from build123d import *

# Parameters (mm, degrees)
SKETCH1_W           = 42.3
SKETCH1_H           = 42.3
SKETCH1_R           = 1.5
SKETCH1_R_2         = 4.7625
BOSS_EXTRUDE1_DEPTH = 5.21
SKETCH2_R           = 0.75565
SKETCH2_R_2         = 1.1303
CUT_EXTRUDE1_DEPTH  = 6.21
CHAMFER1_SIZE       = 2
SKETCH4_R           = 6.96
SKETCH4_R_2         = 4.7625
BOSS_EXTRUDE2_DEPTH = 1.14
SKETCH5_R           = 4
SKETCH5_R_2         = 1.5
CUT_EXTRUDE2_DEPTH  = 2
FILLET1_R           = 5


with BuildPart() as part:
    # Sketch1 → Boss-Extrude1 (new body)
    with BuildSketch(Plane(origin=(0, 0, 0), x_dir=(1, 0, 0), z_dir=(0, 1, 0))):
        with Locations((21.15, 21.15)):
            Rectangle(SKETCH1_W, SKETCH1_H)
        with Locations((36.65, 36.65)):
            Circle(SKETCH1_R, mode=Mode.SUBTRACT)
        with Locations((5.65, 5.65)):
            Circle(SKETCH1_R, mode=Mode.SUBTRACT)
        with Locations((36.65, 5.65)):
            Circle(SKETCH1_R, mode=Mode.SUBTRACT)
        with Locations((5.65, 36.65)):
            Circle(SKETCH1_R, mode=Mode.SUBTRACT)
        with Locations((21.15, 21.15)):
            Circle(SKETCH1_R_2, mode=Mode.SUBTRACT)
    extrude(amount=BOSS_EXTRUDE1_DEPTH)

    # Sketch2 → Cut-Extrude1 (cut, through all)
    with BuildSketch(Plane(origin=(0, 5.21, 0), x_dir=(1, 0, 0), z_dir=(0, 1, 0))):
        with Locations((11.056075115, 23.854659021)):
            Circle(SKETCH2_R)
        with Locations((28.539265863, 28.539265863)):
            Circle(SKETCH2_R)
        with Locations((23.854659021, 11.056075115)):
            Circle(SKETCH2_R)
        with Locations((28.539265863, 13.760734137)):
            Circle(SKETCH2_R_2)
        with Locations((13.760734137, 28.539265863)):
            Circle(SKETCH2_R_2)
    extrude(amount=-CUT_EXTRUDE1_DEPTH, mode=Mode.SUBTRACT)

    # Chamfer1
    chamfer1_edges = [part.edges().sort_by_distance(p)[0] for p in [
        (35.15, 5.21, -36.65),
        (4.15, 5.21, -5.65),
        (35.15, 5.21, -5.65),
        (4.15, 5.21, -36.65),
    ]]
    chamfer(chamfer1_edges, length=CHAMFER1_SIZE)

    # Sketch4 → Boss-Extrude2 (add)
    with BuildSketch(Plane(origin=(0, 5.21, 0), x_dir=(1, 0, 0), z_dir=(0, 1, 0))):
        with Locations((21.15, 21.15)):
            Circle(SKETCH4_R)
        with Locations((21.15, 21.15)):
            Circle(SKETCH4_R_2, mode=Mode.SUBTRACT)
    extrude(amount=BOSS_EXTRUDE2_DEPTH)

    # Sketch5 → Cut-Extrude2 (cut)
    with BuildSketch(Plane.XZ):
        with Locations((36.65, -36.65)):
            Circle(SKETCH5_R)
        with Locations((36.65, -36.65)):
            Circle(SKETCH5_R_2, mode=Mode.SUBTRACT)
        with Locations((5.65, -36.65)):
            Circle(SKETCH5_R)
        with Locations((5.65, -36.65)):
            Circle(SKETCH5_R_2, mode=Mode.SUBTRACT)
        with Locations((5.65, -5.65)):
            Circle(SKETCH5_R)
        with Locations((5.65, -5.65)):
            Circle(SKETCH5_R_2, mode=Mode.SUBTRACT)
        with Locations((36.65, -5.65)):
            Circle(SKETCH5_R)
        with Locations((36.65, -5.65)):
            Circle(SKETCH5_R_2, mode=Mode.SUBTRACT)
    extrude(amount=-CUT_EXTRUDE2_DEPTH, mode=Mode.SUBTRACT)

    # Fillet1
    fillet1_edges = [part.edges().sort_by_distance(p)[0] for p in [
        (0, 2.605, -42.3),
        (42.3, 2.605, -42.3),
        (42.3, 2.605, 0),
        (0, 2.605, 0),
    ]]
    fillet(fillet1_edges, radius=FILLET1_R)


solid = part.part
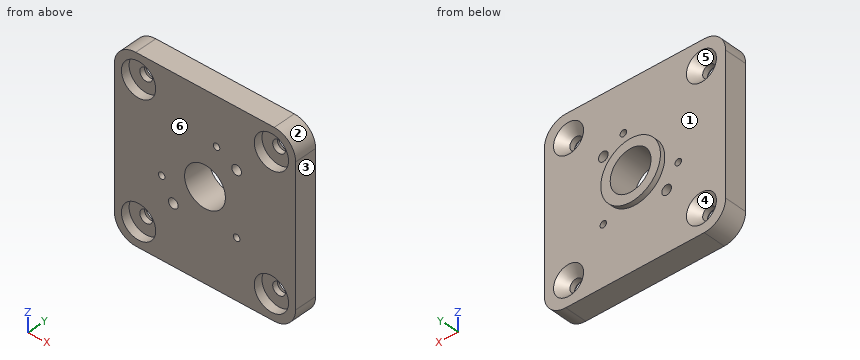
Could you check a few things on this model? Use its own coordinates, in mm. Face numbers are marked on the shaded views. A direction names the side the tool comes from. Give positions to 0.01 mm unless a question says otherwise; leave off trailing zeros. Loops run counter-clockwise (first coordinate to the right, second up) from the corner with the lowest first, then second, coordinate; pieces in that order, holes last. Notation, with made-up numbers: M 78.25,-24 L 104.25,-24 A22 cw 104.25,2 Z; hole C 89.25,40 d7. An arc over 180 degrees is marked long. Answer as a JSON object with one key per item and string values.
Q1. Suppose I cut it at B-B, the plane x = 36.65. List the corners of the cut face in (y, z) for me, plus the area to 3 significant figures.
Values found:
{"outline": "M 0,-42.3 L 5.21,-42.3 L 5.21,-40.15 L 3.21,-38.15 L 2,-38.15 L 2,-40.65 L 0,-40.65 Z; M 0,-32.65 L 2,-32.65 L 2,-35.15 L 3.21,-35.15 L 5.21,-33.15 L 5.21,-9.15 L 3.21,-7.15 L 2,-7.15 L 2,-9.65 L 0,-9.65 Z; M 0,-1.65 L 2,-1.65 L 2,-4.15 L 3.21,-4.15 L 5.21,-2.15 L 5.21,0 L 0,0 Z", "area": "161 mm²"}
Q2. Suppose I cut it at D-D, the plane y = 4.5. State how many separate pieces and enclosed holes the cut face has, plus the area to 3 significant figures.
Values found:
{"separate pieces": "1", "enclosed holes": "10", "area": "1,590 mm²"}
Q3. Suppose I cut it at C-C, the plane z = -5.65. List the corners of the cut face in (x, y) for me, plus the area to 3 significant figures.
Values found:
{"outline": "M 0,0 L 1.65,0 L 1.65,2 L 4.15,2 L 4.15,3.21 L 2.15,5.21 L 0,5.21 Z; M 7.15,2 L 9.65,2 L 9.65,0 L 32.65,0 L 32.65,2 L 35.15,2 L 35.15,3.21 L 33.15,5.21 L 9.15,5.21 L 7.15,3.21 Z; M 38.15,2 L 40.65,2 L 40.65,0 L 42.3,0 L 42.3,5.21 L 40.15,5.21 L 38.15,3.21 Z", "area": "161 mm²"}
Q4. If I drill on probe 1 along Z at (x, y) = (36.65, 2.35); probe 2 along X at (y, z) = (2.5, -36.65); probe 3 along X at (y, z) = (1.25, -33.5), over which ranges is the centre line in solid material (lowest first)? Write a range as [from, to].
Values found:
{"probe 1": "z = [-42.3, -38.15], [-35.15, -7.15], [-4.15, 0]", "probe 2": "x = [0, 4.15], [7.15, 35.15], [38.15, 42.3]", "probe 3": "x = [0, 3.18], [8.12, 34.18], [39.12, 42.3]"}
Q5. For the marked faces 1 and 2, which set-ups out of +Z, -Z, +X, -X, +Y, -Y let a thin tool reach every point of the face, with its end or its side?
Values found:
{"face 1": "+Y", "face 2": "+Z, +X, +Y, -Y"}
Q6. For P1, Ø2.5, axis at x = 38, z = -4, coming from the -Y side; P2, Ø10.5, axis at x = 36.65, z = -5.65, coming from the +Y side; P3, Ø1.4, axis at x = 28.54, z = -28.54, coming from the -Y side; P4, Ø5, axis at x = 36.65, z = -5.65, coming from the +Y side, each with a flat end and sliding along its axis, tell me the tip position at first contact or that it passes through.
Values found:
{"P1": "stops at y = 2", "P2": "stops at y = 5.21", "P3": "passes through", "P4": "stops at y = 4.21"}
Q7. If we mould it in two halves opening along X, with no side actions, what happens to the marked faces 3, 4, 5 and 6? For each: pulls with the +X half, pulls with the -X half, needs draft (parallel to the pull), parting line crosses it, or undercut.
Values found:
{"face 3": "pulls with the +X half", "face 4": "undercut", "face 5": "undercut", "face 6": "needs draft"}
Q8. Suppose I cut it at A-A, the plane z = -21.15. List the corners of the cut face in (x, y) for me, plus the area to 3 significant figures.
Values found:
{"outline": "M 0,0 L 16.39,0 L 16.39,6.35 L 14.19,6.35 L 14.19,5.21 L 0,5.21 Z; M 25.91,0 L 42.3,0 L 42.3,5.21 L 28.11,5.21 L 28.11,6.35 L 25.91,6.35 Z", "area": "176 mm²"}
